Autodesk Inventor part; units mm, degrees
ref_plane "YZ Plane" through (0, 0, 0) normal (1, 0, 0) x (0, 1, 0)
ref_plane "XZ Plane" through (0, 0, 0) normal (0, 1, 0) x (-1, 0, 0)
ref_plane "XY Plane" through (0, 0, 0) normal (0, 0, 1) x (1, 0, 0)
sketch "Sketch1" plane through (0, 0, 0) normal (0, 1, 0) x (-1, 0, 0)
  line L0 (25, 40) -> (-30.5, 40)
  line L1 (-30.5, 40) -> (-30.5, -50)
  line L2 (-30.5, -50) -> (25, -50)
  line L3 (25, -50) -> (25, 40)
  line L4 (25, 40) -> (15, 40)
  line L5 (15, 40) -> (15, 0)
  line L6 (25, -50) -> (25, -40) construction
  line L7 (25, -40) -> (20.5, -40) construction
  line L8 (20.5, -40) -> (20.5, -9) construction
  line L9 (20.5, -9) -> (-10.5, -9) construction
  line L10 (-10.5, -9) -> (-10.5, -40) construction
  line L11 (-10.5, -40) -> (20.5, -40) construction
  circle A0 centre (5, -24.5) radius 12.5
  circle A1 centre (20.5, -9) radius 2
  circle A2 centre (20.5, -40) radius 2
  circle A3 centre (-10.5, -9) radius 2
  circle A4 centre (-10.5, -40) radius 2
  line L12 (15, 40) -> (5, 40) construction
  line L13 (5, 40) -> (5, 30) construction
  line L14 (5, 30) -> (15, 30) construction
  line L15 (15, 30) -> (15, 40) construction
  line L16 (5, 30) -> (-15, 30) construction
  line L17 (-15, 30) -> (-15, 10) construction
  line L18 (-15, 10) -> (5, 10) construction
  line L19 (5, 10) -> (5, 30) construction
  circle A5 centre (5, 30) radius 2.5
  circle A6 centre (5, 10) radius 2.5
  circle A7 centre (-15, 30) radius 2.5
  circle A8 centre (-15, 10) radius 2.5
  line L20 (15, 0) -> (25, 0)
  point P0 (25, -5)
  dimension "d0" = 55.5
  dimension "d1" = 90
  dimension "d2" = 10
  dimension "d3" = 40
  dimension "d4" = 10
  dimension "d5" = 4.5
  dimension "d6" = 31
  dimension "d7" = 31
  dimension "d8" = 31
  dimension "d9" = 25
  dimension "d10" = 4
  dimension "d11" = 4
  dimension "d12" = 4
  dimension "d13" = 4
  dimension "d14" = 10
  dimension "d15" = 10
  dimension "d16" = 20
  dimension "d17" = 20
  dimension "d18" = 5
  dimension "d19" = 5
  dimension "d20" = 5
  dimension "d21" = 5
  dimension "d25" = 15.5
extrude "Extrusion1" add sketch "Sketch1" along normal blind 3 contours L5 L20 L3 L2 L1 L0
sketch "Sketch2" plane through (0, 0, 0) normal (0, -1, 0) x (1, 0, 0)
  line L0 (30.5, 40) -> (30.5, -50)
  line L1 (-25, -50) -> (-25, 0)
  line L2 (30.5, -50) -> (-25, -50)
  line L3 (-25, -50) -> (-25, -47)
  line L4 (-25, -47) -> (30.5, -47)
  line L5 (30.5, -47) -> (30.5, -50)
  point P0 (0, 0)
  dimension "d26" = 3
extrude "Extrusion2" add sketch "Sketch2" along normal blind 35
sketch "Sketch3" plane through (-25, 0, -47) normal (0, 0, 1) x (1, 0, 0)
  line L0 (55.5, -35) -> (55.5, 3) construction
  line L1 (0, 0) -> (0, -35)
  line L2 (10, 3) -> (55.5, 3) construction
  line L3 (55.5, 3) -> (55.5, -17.5) construction
  line L4 (55.5, -17.5) -> (0, -17.5) construction
  line L5 (0, 3) -> (0, -35) construction
  line L6 (55.5, -17.5) -> (40, -17.5) construction
  line L7 (40, -17.5) -> (19.5, -17.5) construction
  line L8 (19.5, -23.5) -> (19.5, -11.5) construction
  line L9 (22.25, -23.5) -> (22.25, -11.5)
  line L10 (16.75, -11.5) -> (16.75, -23.5)
  arc A0 (16.75, -23.5) -> (22.25, -23.5) centre (19.5, -23.5) ccw
  arc A1 (22.25, -11.5) -> (16.75, -11.5) centre (19.5, -11.5) ccw
  line L11 (40, -23.5) -> (40, -11.5) construction
  line L12 (42.75, -23.5) -> (42.75, -11.5)
  line L13 (37.25, -11.5) -> (37.25, -23.5)
  arc A2 (37.25, -23.5) -> (42.75, -23.5) centre (40, -23.5) ccw
  arc A3 (42.75, -11.5) -> (37.25, -11.5) centre (40, -11.5) ccw
  line L14 (10, 0) -> (55.5, 0)
  point P0 (25, 0)
  dimension "d38" = 15.5
  dimension "d39" = 20.5
  dimension "d40" = 6
  dimension "d41" = 5.5
  dimension "d42" = 6
  dimension "d43" = 5.5
  dimension "d47" = 17.5
extrude "Extrusion3" cut sketch "Sketch3" against normal through all
fillet "Fillet3" radius 10 4 edges at (-25, 1.5, 0) (-15, 1.5, 40) (30.5, 1.5, 40) (-15, 1.5, 0)
fillet "Fillet4" radius 25 2 edges at (-25, -35, -48.5) (30.5, -35, -48.5)
properties part number "ActuatorPulleyPlate" material "Aluminum 6061"
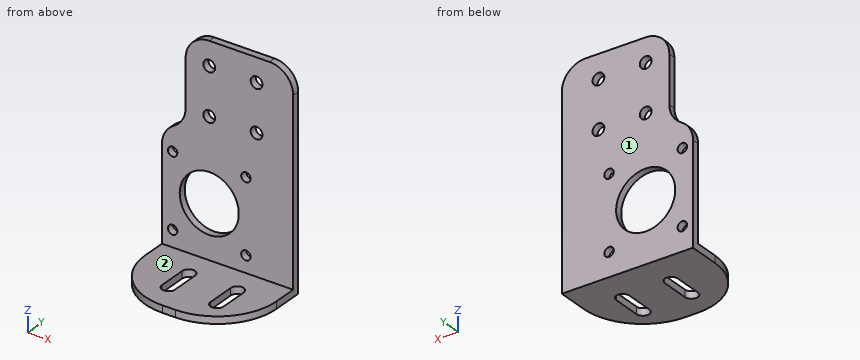
Work out the finished part from the listing and answer in its coordinate system (mm). Face numbers are marked on the shaded views. A direction names the side the tool comes from. Give positions to 0.01 mm unless a question says otherwise; leave off trailing zeros. Loops run counter-clockwise (first coordinate to the right, second up) from the corner with the lowest first, then second, coordinate; pieces in that order, holes last. Notation, with made-up numbers: (3, -32) -> (53, -32) arc R16 cw to (53, -2) -> close; hole circle Ø7 at (28, 46). An arc over 180 degrees is marked (long way). Use a Markdown table: item, result. Add a question column.
1) Each of these flat-tipped pins is pushed along its axis until it touches: P1, Ø8, axis at x = 15, z = 10, coming from the -Y side; P2, Ø2.5, axis at y = 1.5, z = 18, coming from the -X side; P3, Ø1.5, axis at y = -18, z = -48.5, coming from the +X side. Where does it stop, or does it pass through?
2) Consider line 1 along Z through (x, y) = (-5, 2); line 2 along X through (y, z) = (1.5, 10.5); line 3 along Z through (x, y) = (10.5, 2.2). Determine where each line is inside the solid, lowest interval first.
3) The part is cut by section C-C, the plane x = 15. Determine the outline of the cut face in (y, z).
4) The part is cut by section B-B, the plane x = 3. Determine the outline of the cut face in (y, z), plus the area to 3 significant figures.
5) The part is cut by section A-A, the plane z = -24.5. Determine the outline of the cut face in (x, y).
6) The part is cut by section D-D, the plane z = -10. Determine the outline of the cut face in (x, y), plus the area to 3 significant figures.
7) Which of the six approach directions +Z, -Z, +X, -X, +Y, -Y give full straight-line access (tool end or side, diameter ignored) to the marked faces 1 and 2?
Reported:
| question | item | result |
|---|---|---|
| 1 | P1 | stops at y = 0 |
| 1 | P2 | stops at x = -15 |
| 1 | P3 | stops at x = 29.43 |
| 2 | line 1 | z = -50 to -37, -12 to 7.5, 12.5 to 27.5, 32.5 to 40 |
| 2 | line 2 | x = -15 to -7.45, -2.55 to 12.55, 17.45 to 30.5 |
| 2 | line 3 | z = -50 to -42, -38 to -11, -7 to 40 |
| 3 | outline | (-33.12, -50) -> (-26.25, -50) -> (-26.25, -47) -> (-33.12, -47) -> close; (-8.75, -50) -> (3, -50) -> (3, 7.5) -> (0, 7.5) -> (0, -47) -> (-8.75, -47) -> close; (0, 12.5) -> (3, 12.5) -> (3, 27.5) -> (0, 27.5) -> close; (0, 32.5) -> (3, 32.5) -> (3, 40) -> (0, 40) -> close |
| 4 | outline | (-35, -50) -> (3, -50) -> (3, -34.1) -> (0, -34.1) -> (0, -47) -> (-35, -47) -> close; (0, -14.9) -> (3, -14.9) -> (3, 40) -> (0, 40) -> close |
| 4 | area | 317 mm^2 |
| 5 | outline | (-25, 0) -> (-17.5, 0) -> (-17.5, 3) -> (-25, 3) -> close; (7.5, 0) -> (30.5, 0) -> (30.5, 3) -> (7.5, 3) -> close |
| 6 | outline | (-25, 0) -> (-22.23, 0) -> (-22.23, 3) -> (-25, 3) -> close; (-18.77, 0) -> (8.77, 0) -> (8.77, 3) -> (-18.77, 3) -> close; (12.23, 0) -> (30.5, 0) -> (30.5, 3) -> (12.23, 3) -> close |
| 6 | area | 146 mm^2 |
| 7 | face 1 | +Z, -Z, +X, -X, +Y |
| 7 | face 2 | +Z, +X, -X, -Y |
